from build123d import *

# Parameters (mm, degrees)
SKETCH1_W           = 72
SKETCH1_H           = 92
BOSS_EXTRUDE1_DEPTH = 3
SKETCH2_W           = 5
SKETCH2_H           = 92
BOSS_EXTRUDE2_DEPTH = 47
BOSS_EXTRUDE3_REACH = 52
SKETCH3_W           = 52
SKETCH3_H           = 20
CUT_EXTRUDE3_REACH  = 54
SKETCH8_W           = 52
SKETCH8_H           = 16.552945357
BOSS_EXTRUDE5_DEPTH = 2
SKETCH9_W           = 52
SKETCH9_H           = 5
SKETCH9_H_2         = 0.845770931
BOSS_EXTRUDE6_DEPTH = 1.812366
SKETCH10_W          = 42
SKETCH10_H          = 40
CUT_EXTRUDE4_DEPTH  = 17
CUT_EXTRUDE5_REACH  = 94
SKETCH12_R          = 1.5
SKETCH13_W          = 72
SKETCH13_H          = 3
BOSS_EXTRUDE7_DEPTH = 20
SKETCH15_W          = 3
SKETCH15_H          = 112
BOSS_EXTRUDE8_DEPTH = 20
SKETCH16_W          = 3
SKETCH16_H          = 112
BOSS_EXTRUDE9_DEPTH = 42
CUT_EXTRUDE9_REACH  = 5
SKETCH14_R          = 1.5


with BuildPart() as part:
    # Sketch1 → Boss-Extrude1 (new body)
    with BuildSketch(Plane.XY):
        Rectangle(SKETCH1_W, SKETCH1_H)
    extrude(amount=BOSS_EXTRUDE1_DEPTH)

    # Sketch2 → Boss-Extrude2 (add)
    with BuildSketch(Plane.XY.offset(3)):
        with Locations((33.5, 0)):
            Rectangle(SKETCH2_W, SKETCH2_H)
        with Locations((-13.5, 0)):
            Rectangle(SKETCH2_W, SKETCH2_H)
    extrude(amount=BOSS_EXTRUDE2_DEPTH)

    # Sketch3 → Boss-Extrude3 (add, up to next)
    with BuildSketch(Plane.XY.offset(50), mode=Mode.PRIVATE) as boss_extrude3_sk1:
        with Locations((10, 36)):
            Rectangle(SKETCH3_W, SKETCH3_H)
    boss_extrude3_tool1 = extrude(boss_extrude3_sk1.sketch, amount=-BOSS_EXTRUDE3_REACH, mode=Mode.PRIVATE) - part.part
    add(boss_extrude3_tool1.solids().sort_by_distance((10, 36, 50))[0])

    # Sketch7 → Cut-Extrude3 (cut, up to next)
    with BuildSketch(Plane.ZY.offset(16), mode=Mode.PRIVATE) as cut_extrude3_sk1:
        Polygon((50, 41), (15, -34), (15, -46), (50, -46), align=None)
    cut_extrude3_tool1 = extrude(cut_extrude3_sk1.sketch, amount=-CUT_EXTRUDE3_REACH, mode=Mode.PRIVATE) & part.part
    add(cut_extrude3_tool1.solids().sort_by_distance((-16, -16.515152, 36.919192))[0], mode=Mode.SUBTRACT)

    # Sketch8 → Boss-Extrude5 (add)
    with BuildSketch(Plane(origin=(0, -11.828467153, 25.346715328), x_dir=(1, 0, 0), z_dir=(0, -0.422885465, 0.90618314))):
        with Locations((10, 50.021309328)):
            Rectangle(SKETCH8_W, SKETCH8_H)
    extrude(amount=BOSS_EXTRUDE5_DEPTH)

    # Sketch9 → Boss-Extrude6 (add)
    with BuildSketch(Plane.XY.offset(50)):
        with Locations((10, 43.5)):
            Rectangle(SKETCH9_W, SKETCH9_H)
        with Locations((10, 40.577114534)):
            Rectangle(SKETCH9_W, SKETCH9_H_2)
    extrude(amount=BOSS_EXTRUDE6_DEPTH)

    # Sketch10 → Cut-Extrude4 (cut)
    with BuildSketch(Plane.XZ.offset(-26)):
        with Locations((10, 23)):
            Rectangle(SKETCH10_W, SKETCH10_H)
    extrude(amount=-CUT_EXTRUDE4_DEPTH, mode=Mode.SUBTRACT)

    # Sketch12 → Cut-Extrude5 (cut, up to next)
    with BuildSketch(Plane(origin=(0, 46, 0), x_dir=(1, 0, 0), z_dir=(0, 1, 0)), mode=Mode.PRIVATE) as cut_extrude5_sk1:
        with Locations((4, -31.81236628)):
            Circle(SKETCH12_R)
    cut_extrude5_tool1 = extrude(cut_extrude5_sk1.sketch, amount=-CUT_EXTRUDE5_REACH, mode=Mode.PRIVATE) & part.part
    add(cut_extrude5_tool1.solids().sort_by_distance((4, 46, 31.812366))[0], mode=Mode.SUBTRACT)
    # Sketch12 → Cut-Extrude5 (cut, up to next)
    with BuildSketch(Plane(origin=(0, 46, 0), x_dir=(1, 0, 0), z_dir=(0, 1, 0)), mode=Mode.PRIVATE) as cut_extrude5_sk2:
        with Locations((19, -31.81236628)):
            Circle(SKETCH12_R)
    cut_extrude5_tool2 = extrude(cut_extrude5_sk2.sketch, amount=-CUT_EXTRUDE5_REACH, mode=Mode.PRIVATE) & part.part
    add(cut_extrude5_tool2.solids().sort_by_distance((19, 46, 31.812366))[0], mode=Mode.SUBTRACT)

    # Sketch13 → Boss-Extrude7 (add)
    with BuildSketch(Plane(origin=(0, 46, 0), x_dir=(1, 0, 0), z_dir=(0, 1, 0))):
        with Locations((0, -1.5)):
            Rectangle(SKETCH13_W, SKETCH13_H)
    extrude(amount=BOSS_EXTRUDE7_DEPTH)

    # Sketch15 → Boss-Extrude8 (add)
    with BuildSketch(Plane(origin=(36, 0, 0), x_dir=(0, 0, -1), z_dir=(1, 0, 0))):
        with Locations((-1.5, 10)):
            Rectangle(SKETCH15_W, SKETCH15_H)
    extrude(amount=BOSS_EXTRUDE8_DEPTH)

    # Sketch16 → Boss-Extrude9 (add)
    with BuildSketch(Plane.ZY.offset(36)):
        with Locations((1.5, 10)):
            Rectangle(SKETCH16_W, SKETCH16_H)
    extrude(amount=BOSS_EXTRUDE9_DEPTH)

    # Sketch14 → Cut-Extrude9 (cut, up to next)
    with BuildSketch(Plane.XY.offset(3), mode=Mode.PRIVATE) as cut_extrude9_sk1:
        with Locations((24, 56)):
            Circle(SKETCH14_R)
    cut_extrude9_tool1 = extrude(cut_extrude9_sk1.sketch, amount=-CUT_EXTRUDE9_REACH, mode=Mode.PRIVATE) & part.part
    add(cut_extrude9_tool1.solids().sort_by_distance((24, 56, 3))[0], mode=Mode.SUBTRACT)
    # Sketch14 → Cut-Extrude9 (cut, up to next)
    with BuildSketch(Plane.XY.offset(3), mode=Mode.PRIVATE) as cut_extrude9_sk2:
        with Locations((10, -36)):
            Circle(SKETCH14_R)
    cut_extrude9_tool2 = extrude(cut_extrude9_sk2.sketch, amount=-CUT_EXTRUDE9_REACH, mode=Mode.PRIVATE) & part.part
    add(cut_extrude9_tool2.solids().sort_by_distance((10, -36, 3))[0], mode=Mode.SUBTRACT)
    # Sketch14 → Cut-Extrude9 (cut, up to next)
    with BuildSketch(Plane.XY.offset(3), mode=Mode.PRIVATE) as cut_extrude9_sk3:
        with Locations((-66, 56)):
            Circle(SKETCH14_R)
    cut_extrude9_tool3 = extrude(cut_extrude9_sk3.sketch, amount=-CUT_EXTRUDE9_REACH, mode=Mode.PRIVATE) & part.part
    add(cut_extrude9_tool3.solids().sort_by_distance((-66, 56, 3))[0], mode=Mode.SUBTRACT)


solid = part.part
The listing builds one solid part. Answer for the finished solid, in the listing's coordinates (mm). A direction names the side the tool comes from. Give positions to 0.01 mm unless a question says otherwise; leave off trailing zeros. Order: outer loops, then holes, each group sorted by start corner. A loop starts at its lowest first (then second) coordinate and runs counter-clockwise, first axis right, second up. Notation, with made-up numbers: (3.25, 63.25) - (8.25, 63.25) arc R13 cw to (8.25, 80.25) - close; hole circle Ø5 at (-1.5, 7.25). An arc over 180 degrees is marked (long way). Answer as CSV lines item,"result".
Q1. Straight lines are drawn through the part: L1, parallel to Z at x = 4, y = 42.5; L2, parallel to X at y = 41.5, z = 20; L3, parallel to Z at x = 19, y = 44. For each, find the intervals that lie inside material, in ascending order.
Answer key:
L1,"z = 0 to 3, 43 to 51.81"
L2,"x = -16 to -11, 31 to 36"
L3,"z = 0 to 30.31, 33.31 to 51.81"
Q2. A cutting plane is placed at D-D, the plane z = 36.5. Determine the outline of the cut face in (x, y), and give its area (3 significant figures).
Answer key:
outline,"(-16, 12.07) - (-11, 12.07) - (-11, 43) - (31, 43) - (31, 12.07) - (36, 12.07) - (36, 46) - (-16, 46) - close"
area,"465 mm^2"
Q3. Which of the six approach directions +Z, -Z, +X, -X, +Y, -Y give full straight-line access (tool end or side, diameter ignored) to faces 1 (the face through (10, 46, 27)), 2 (the face through (-25, 22, 3)), 3 (the face through (10, -1, 3))?
Answer key:
face 1,"+Z, +X, -X, +Y"
face 2,"+Z, +Y"
face 3,"-Y"
Q4. A cutting plane is placed at C-C, the plane y = 18.5. Determine the outline of the cut face in (x, z), and give its area (3 significant figures).
Answer key:
outline,"(-78, 0) - (56, 0) - (56, 3) - (36, 3) - (36, 39.5) - (31, 39.5) - (31, 3) - (-11, 3) - (-11, 39.5) - (-16, 39.5) - (-16, 3) - (-78, 3) - close"
area,"767 mm^2"
Q5. A cutting plane is placed at B-B, the plane y = 56. Determine the outline of the cut face in (x, z).
Answer key:
outline,"(-78, 0) - (-67.5, 0) - (-67.5, 3) - (-78, 3) - close; (-64.5, 0) - (22.5, 0) - (22.5, 3) - (-64.5, 3) - close; (25.5, 0) - (56, 0) - (56, 3) - (25.5, 3) - close"
Q6. A cutting plane is placed at A-A, the plane x = 19. Determine the outline of the cut face in (y, z), and give its area (3 significant figures).
Answer key:
outline,"(-46, 0) - (66, 0) - (66, 3) - (46, 3) - (46, 30.31) - (43, 30.31) - (43, 3) - (-46, 3) - close; (25.15, 44.81) - (26, 43) - (43, 43) - (43, 33.31) - (46, 33.31) - (46, 51.81) - (40.15, 51.81) - close"
area,"577 mm^2"
Q7. Each of these flat-tipped pins is pushed along its axis until it touches: pin 1 Ø3 at (x, z) = (-3.5, 33.5) entering from -Y; pin 2 Ø14.5 at (x, z) = (15.5, 30) entering from +Y; pin 3 Ø1.5 at (x, y) = (-13, -38) entering from +Z; pin 4 Ø2.5 at (x, z) = (19, 31.81) entering from -Y. Where does it stop, or does it pass through?
Answer key:
pin 1,"stops at y = 43"
pin 2,"stops at y = 46"
pin 3,"stops at z = 15"
pin 4,"passes through"
Q8. Determine the mould class of faces 4 (the face through (-16, 11, 22)), 5 (the face through (33, -40, 15)), 6 (the face through (10, 34, 43)) for opening direction Z: pulls with the +Z half, pulls with the -Z half, needs draft (parallel to the pull), parting line crosses it, or undercut.
Answer key:
face 4,"needs draft"
face 5,"pulls with the +Z half"
face 6,"undercut"
